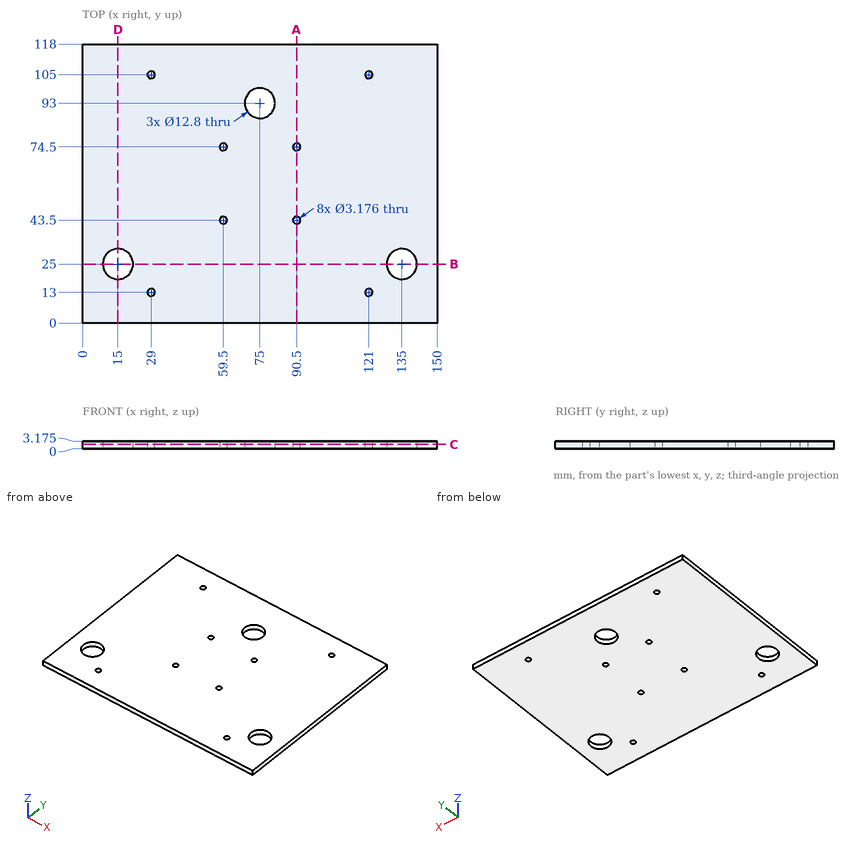
Geometry check sheet. Reference: drawing and pictorial views, mm from the part's lowest x, y, z. Give positions to 0.01 mm unless a question says otherwise; leave off trailing zeros. Write each loop counter-clockwise with the first axis right and the second up, starting at its lowest first coordinate (ties: lowest second). Pieces come first, ordered by that corner, then holes. Notation, with made-up numbers: (79, -37.5) -> (128, -37.5) arc R26 ccw to (128, -8.5) -> close; hole circle Ø10 at (72.25, 2.25). An arc over 180 degrees is marked (long way). One line per item, written item: value. Start each with the question number.
Item 1: Section check C-C on z = 1.85. State how many separate pieces and enclosed holes the cut face has, then the cut area to 3 significant figures.
Item 2: Material ranges on probe 1 along Y at (x, z) = (90.5, 2.4); probe 2 along Y at (x, z) = (121, 2.5); probe 3 along X at (y, z) = (105, 1.2), recorded low to high. Write a range as from..to.
Item 3: Section check D-D on x = 15. Record the cut outline in (y, z) (3 decimals), then the cut area to 3 significant figures.
Item 4: Section check B-B on y = 25. Record the cut outline in (x, z) (3 decimals).
Item 5: Gauge pin test, flat end, axial feed: pin 1 (10 mm diameter, centred on x = 75, y = 93, fed in from -Z). Record the tip position at first contact, or that the pin passes through.
Item 6: Section check A-A on x = 90.5. Record the cut outline in (y, z) (3 decimals).
Results list:
1. separate pieces: 1
1. enclosed holes: 11
1. area: 17,300 mm²
2. probe 1: 0..41.91, 45.09..72.91, 76.09..118
2. probe 2: 0..11.41, 14.59..103.41, 106.59..118
2. probe 3: 0..27.41, 30.59..119.41, 122.59..150
3. outline: (0, 0) -> (18.6, 0) -> (18.6, 3.175) -> (0, 3.175) -> close; (31.4, 0) -> (118, 0) -> (118, 3.175) -> (31.4, 3.175) -> close
3. area: 334 mm²
4. outline: (0, 0) -> (8.6, 0) -> (8.6, 3.175) -> (0, 3.175) -> close; (21.4, 0) -> (128.6, 0) -> (128.6, 3.175) -> (21.4, 3.175) -> close; (141.4, 0) -> (150, 0) -> (150, 3.175) -> (141.4, 3.175) -> close
5. pin 1: through
6. outline: (0, 0) -> (41.912, 0) -> (41.912, 3.175) -> (0, 3.175) -> close; (45.088, 0) -> (72.912, 0) -> (72.912, 3.175) -> (45.088, 3.175) -> close; (76.088, 0) -> (118, 0) -> (118, 3.175) -> (76.088, 3.175) -> close
